from build123d import *

# Parameters (mm, degrees)
RESSALTO_EXTRUS_O1_DEPTH = 1.5
ESBO_O2_R                = 1.65
CORTE_EXTRUS_O1_DEPTH    = 100.040395799


with BuildPart() as part:
    # Esboço1 → Ressalto-extrusão1 (new, symmetric)
    with BuildSketch(Plane(origin=(0, 0, 0), x_dir=(1, 0, 0), z_dir=(0, 1, 0))):
        Polygon((70, 28.994949366), (28.994949366, 70), (-28.994949366, 70), (-70, 28.994949366), (-70, -28.994949366), (-28.994949366, -70), (28.994949366, -70), (70, -28.994949366), align=None)
    extrude(amount=RESSALTO_EXTRUS_O1_DEPTH, both=True)

    # Esboço2 → Corte-extrusão1 (cut, through all)
    with BuildSketch(Plane.XZ.offset(1.5)):
        with Locations(Location((-26.31616534, 63.532843272, 0), (0, 0, 270))):
            Circle(ESBO_O2_R)
        with Locations(Location((26.31616534, 63.532843272, 0), (0, 0, 270))):
            Circle(ESBO_O2_R)
        with Locations(Location((63.532843272, 26.31616534, 0), (0, 0, 270))):
            Circle(ESBO_O2_R)
        with Locations(Location((63.532843272, -26.31616534, 0), (0, 0, 270))):
            Circle(ESBO_O2_R)
        with Locations(Location((26.31616534, -63.532843272, 0), (0, 0, 270))):
            Circle(ESBO_O2_R)
        with Locations(Location((-26.31616534, -63.532843272, 0), (0, 0, 270))):
            Circle(ESBO_O2_R)
        with Locations(Location((-63.532843272, 26.31616534, 0), (0, 0, 270))):
            Circle(ESBO_O2_R)
        with Locations(Location((-63.532843272, -26.31616534, 0), (0, 0, 270))):
            Circle(ESBO_O2_R)
    extrude(amount=-CORTE_EXTRUS_O1_DEPTH, mode=Mode.SUBTRACT)


solid = part.part
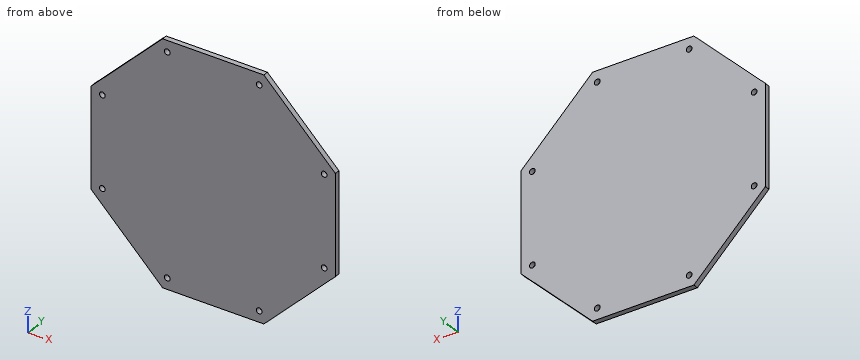
Work out the finished part from the listing and answer in its coordinate system (mm). Give positions to 0.01 mm unless a question says otherwise; leave off trailing zeros. Order: outer loops, then holes, each group sorted by start corner. A loop starts at its lowest first (then second) coordinate and runs counter-clockwise, first axis right, second up. Notation, with made-up numbers: (83, 51) -> (101, 51) arc R19 ccw to (101, 57) -> close; hole circle Ø6 at (-18.5, 74). An arc over 180 degrees is marked (long way). One line per item, written item: value.
Item 1: Find section B-B, the plane z = -60. Give the vertices of the cut face in (x, y), plus the area to 3 significant figures.
Answer sheet:
outline: (-38.99, -1.5) -> (38.99, -1.5) -> (38.99, 1.5) -> (-38.99, 1.5) -> close
area: 234 mm²
Item 2: Straight lines are drawn through the part: probe 1 along Z at (x, y) = (-25, -0.5); probe 2 along X at (y, z) = (0.85, 64); probe 3 along Z at (x, y) = (-56.5, -1.1). For each, find the intervals that lie inside material, in ascending order.
Answer sheet:
probe 1: -70 to -64.53, -62.54 to 62.54, 64.53 to 70
probe 2: -34.99 to -27.9, -24.73 to 24.73, 27.9 to 34.99
probe 3: -42.49 to 42.49
Item 3: Find section C-C, the plane x = 43. Give the vertices of the cut face in (y, z).
Answer sheet:
outline: (-1.5, -55.99) -> (1.5, -55.99) -> (1.5, 55.99) -> (-1.5, 55.99) -> close
Item 4: Flat-ended cylindrical pins translate along their axes: P1, Ø1, axis at y = 0, z = -30.5, coming from the +X side; P2, Ø4, axis at x = 63.53, z = -26.32, coming from the -Y side. Find the tip coordinate at first contact, or state that the pin passes through.
Answer sheet:
P1: x = 68.99
P2: y = -1.5
Item 5: Find section A-A, the plane y = -0.95. State how many separate pieces and enclosed holes the cut face has, plus the area to 3 significant figures.
Answer sheet:
separate pieces: 1
enclosed holes: 8
area: 16,200 mm²
